Could you check a few things on this model? Use its own coordinates, in mm. A direction names the side the tool comes from. Give positions to 0.01 mm unless a question says otherwise; leave off trailing zeros. Order: outer loops, then holes, each group sorted by start corner. A loop starts at its lowest first (then second) coordinate and runs counter-clockwise, first axis right, second up. Notation, with made-up numbers: (-23, -18.5) -> (-7, -18.5) arc R24 ccw to (-7, 5.5) -> close; hole circle Ø9 at (9, 24). An arc over 180 degrees is marked (long way). Write each question's results on one line, items separated by ' | '.
Solid Edge part; units mm, degrees
sketch "Sketch1" plane through (0, 0, 0) normal (0, -1, 0) x (1, 0, 0)
  line L0 (-20, -20) -> (20, -20)
  line L1 (20, -20) -> (20, 20)
  line L2 (20, 20) -> (-20, 20)
  line L3 (-20, 20) -> (-20, -20)
extrude "Protrusion1" add sketch "Sketch1" along normal mid plane 9
sketch "Sketch2" plane through (0, -4.5, 0) normal (0, -1, 0) x (1, 0, 0)
  line L0 (-15.3, -15.3) -> (15.3, -15.3)
  line L1 (15.3, -15.3) -> (15.3, -9)
  line L2 (10.3, -4) -> (15.3, -9)
  line L3 (10.3, 4) -> (10.3, -4)
  line L4 (10.3, 4) -> (15.3, 9)
  line L5 (15.3, 9) -> (15.3, 15.3)
  line L6 (15.3, 15.3) -> (-15.3, 15.3)
  line L7 (-15.3, 15.3) -> (-15.3, 9)
  line L8 (-10.3, 4) -> (-15.3, 9)
  line L9 (-10.3, 4) -> (-10.3, -4)
  line L10 (-10.3, -4) -> (-15.3, -9)
  line L11 (-15.3, -9) -> (-15.3, -15.3)
extrude "ExtrudedCutout_1" cut sketch "Sketch2" against normal blind 161.5
sketch "Sketch3" plane through (0, -21.5, 0) normal (0, -1, 0) x (0, 0, 1)
  line L0 (54.5, -22.5) -> (54.5, 22.5)
  line L1 (54.5, 22.5) -> (9.5, 22.5)
  line L2 (9.5, 22.5) -> (9.5, -22.5)
  line L3 (9.5, -22.5) -> (54.5, -22.5)
extrude "ExtrudedProtrusion_8" add sketch "Sketch3" along normal blind 30
sketch "Sketch4" plane through (0, -36.5, 32) normal (0, -1, 0) x (1, 0, 0)
  line L0 (-21.15, -21.15) -> (21.15, -21.15)
  line L1 (21.15, -21.15) -> (21.15, 21.15)
  line L2 (21.15, 21.15) -> (-21.15, 21.15)
  line L3 (-21.15, 21.15) -> (-21.15, -21.15)
extrude "ExtrudedCutout_4" cut sketch "Sketch4" against normal blind 13 and the other way blind 20
sketch "Sketch5" plane through (0, -23.5, 32) normal (0, -1, 0) x (0, 0, 1)
  circle A0 centre (0, 0) radius 11.5
  circle A1 centre (-15.5, 15.5) radius 1.75
  circle A2 centre (-15.5, -15.5) radius 1.75
  circle A3 centre (15.5, 15.5) radius 1.75
  circle A4 centre (15.5, -15.5) radius 1.75
extrude "Cutout1" cut sketch "Sketch5" against normal up to next
sketch "Sketch6" plane through (0, -4.5, 0) normal (0, -1, 0) x (1, 0, 0)
  line L0 (-20, 20) -> (20, 20)
  line L1 (20, 20) -> (20, -20)
  line L2 (20, -20) -> (-20, -20)
  line L3 (-20, -20) -> (-20, 20)
extrude "ExtrudedProtrusion_9" add sketch "Sketch6" along normal blind 2
sketch "Sketch7" plane through (0, -36.5, 9.5) normal (0, 0, -1) x (1, 0, 0)
  line L0 (-22.5, 15) -> (-22.5, -15)
  line L1 (-22.5, -15) -> (-5.5, -15)
  line L2 (-5.5, -15) -> (-5.5, 15)
  line L3 (-5.5, 15) -> (-22.5, 15)
  line L4 (22.5, 15) -> (22.5, -15)
  line L5 (22.5, -15) -> (5.5, -15)
  line L6 (5.5, -15) -> (5.5, 15)
  line L7 (5.5, 15) -> (22.5, 15)
extrude "ExtrudedProtrusion_13" add sketch "Sketch7" along normal blind 29
sketch "Sketch8" plane through (0, -1, -20) normal (0, 0, -1) x (0, -1, 0)
  line L0 (50.5, 22.5) -> (-5.5, 22.5)
  line L1 (-5.5, 22.5) -> (-5.5, -22.5)
  line L2 (-5.5, -22.5) -> (50.5, -22.5)
  line L3 (50.5, -22.5) -> (50.5, 22.5)
extrude "ExtrudedProtrusion_14" add sketch "Sketch8" against normal blind 4.7
sketch "Sketch9" plane through (0, -23.5, -20) normal (0, 0, -1) x (-1, 0, 0)
  line L0 (-22.5, -28) -> (22.5, -28)
  line L1 (22.5, -28) -> (22.5, 28)
  line L2 (22.5, 28) -> (-22.5, 28)
  line L3 (-22.5, 28) -> (-22.5, -28)
extrude "ExtrudedCutout_6" cut sketch "Sketch9" against normal blind 2.7
sketch "Sketch10" plane through (0, -23.5, -17.3) normal (0, 0, -1) x (-1, 0, 0)
  line L0 (20, 28) -> (22.5, 28)
  line L1 (22.5, 28) -> (22.5, -17)
  line L2 (22.5, -17) -> (-22.5, -17)
  line L3 (-22.5, -17) -> (-22.5, 28)
  line L4 (-22.5, 28) -> (-20, 28)
  line L5 (-20, -12) -> (-20, 28)
  line L6 (20, -12) -> (-20, -12)
  line L7 (20, 28) -> (20, -12)
extrude "ExtrudedProtrusion_15" add sketch "Sketch10" along normal blind 30
Q1. I need wall thicknesses on line 1 along Z through (x, y) = (0, -22.5); line 2 along X through (y, z) = (-22.6, 47.5); line 3 along X through (y, z) = (-41, 19.5). Which ranges of each line are inside material? Lowest first, please.
Here are the results:
line 1: z = -17.3 to -15.3, 9.5 to 20.5, 43.5 to 54.5 | line 2: x = -22.5 to -17.25, -13.75 to 13.75, 17.25 to 22.5 | line 3: x = -22.5 to -21.15, 21.15 to 22.5
Q2. I'm going to push flat-ended pins straight in: pin 1 Ø12 at (x, y) = (-1.5, -25) entering from -Z; pin 2 Ø14 at (x, z) = (0, 32) entering from +Y; pin 3 Ø1.9 at (y, z) = (-1.5, 12.5) entering from -X; pin 4 Ø3.5 at (y, z) = (1, 11) entering from +X. Where does each tip first touch, or does it pass through?
Here are the results:
pin 1: stops at z = -17.3 | pin 2: passes through | pin 3: stops at x = -20 | pin 4: stops at x = 20
Q3. Suppose I cut it at B-B on z = 16.5. Please give me the cut outline in (x, y).
Here are the results:
outline: (-22.5, -51.5) -> (-21.15, -51.5) -> (-21.15, -23.5) -> (-17.25, -23.5) -> (-17.25, -21.5) -> (-22.5, -21.5) -> close; (-20, -6.5) -> (20, -6.5) -> (20, 4.5) -> (-20, 4.5) -> close; (-13.75, -23.5) -> (13.75, -23.5) -> (13.75, -21.5) -> (-13.75, -21.5) -> close; (17.25, -23.5) -> (21.15, -23.5) -> (21.15, -51.5) -> (22.5, -51.5) -> (22.5, -21.5) -> (17.25, -21.5) -> close
Q4. Suppose I cut it at C-C on x = 0. Please give me the cut outline in (y, z).
Here are the results:
outline: (-51.5, -17.3) -> (-40.5, -17.3) -> (-40.5, -47.3) -> (-35.5, -47.3) -> (-35.5, -17.3) -> (4.5, -17.3) -> (4.5, -15.3) -> (-4.5, -15.3) -> (-4.5, 15.3) -> (4.5, 15.3) -> (4.5, 20) -> (-6.5, 20) -> (-6.5, -15.3) -> (-51.5, -15.3) -> close; (-51.5, 9.5) -> (-21.5, 9.5) -> (-21.5, 20.5) -> (-23.5, 20.5) -> (-23.5, 10.85) -> (-51.5, 10.85) -> close; (-51.5, 53.15) -> (-23.5, 53.15) -> (-23.5, 43.5) -> (-21.5, 43.5) -> (-21.5, 54.5) -> (-51.5, 54.5) -> close
Q5. Thinking about a two-plate mould opening in Z: for faces 1 (the flat face through (0, -35.5, -32)), 2 (the flat face through (-9, -23.5, 23)), 3 (the flat face through (0, -1, 20)), which applies, +Z half, -Z half, draft (parallel to the pull), parting line (faces both ways), or undercut?
Here are the results:
face 1: draft | face 2: undercut | face 3: +Z half
Q6. For faces 4 (the flat face through (0, -6.5, 2)), 5 (the flat face through (0, -38, 53.15)), 6 (the flat face through (12.8, -0.1, -6.5)), which set-ups out of +Z, -Z, +X, -X, +Y, -Y let a thin tool reach every point of the face, with its end or its side?
Here are the results:
face 4: +Z, +X, -X | face 5: -Y | face 6: +Y
Q7. Suppose I cut it at A-A on z = 32. Please give me the cut outline in (x, y).
Here are the results:
outline: (-22.5, -51.5) -> (-21.15, -51.5) -> (-21.15, -23.5) -> (-11.5, -23.5) -> (-11.5, -21.5) -> (-22.5, -21.5) -> close; (11.5, -23.5) -> (21.15, -23.5) -> (21.15, -51.5) -> (22.5, -51.5) -> (22.5, -21.5) -> (11.5, -21.5) -> close
Q8. Suppose I cut it at D-D on y = -19. Please give me the cut outline in (x, z), and give its area (3 significant figures).
Here are the results:
outline: (-22.5, -47.3) -> (-20, -47.3) -> (-20, -17.3) -> (20, -17.3) -> (20, -47.3) -> (22.5, -47.3) -> (22.5, -15.3) -> (-22.5, -15.3) -> close | area: 240 mm²
